Design review of the part built by this model. Coordinates are the model's own, in mm. Give positions to 0.01 mm unless a question says otherwise; leave off trailing zeros. Loops run counter-clockwise (first coordinate to the right, second up) from the corner with the lowest first, then second, coordinate; pieces in that order, holes last. Notation, with made-up numbers: M 17,36 L 57,36 A20 ccw 57,65 Z; hole C 28,-15 d9. An arc over 180 degrees is marked long. Use a Markdown table: item, result. Add a question column.
(1) Add section A-A, the plane x = -54.5. Give the boundary of the cut face in (y, z), then the cut area to 3 significant figures.
(2) Add section D-D, the plane x = -22. Give the boundary of the cut face in (y, z), then the cut area to 3 significant figures.
(3) Insertion check: pin 1 Ø0.9 at (y, z) = (-124.5, 2) entering from +X; pin 2 Ø0.9 at (x, z) = (-56, 2) entering from +Y; pin 3 Ø1.5 at (x, z) = (-42, 2) entering from -Y. Each pin has a flat end and moves straight along its axis. Give the tip position at first contact, or say it passes through.
(4) For probe 1 along Y at (x, z) = (16.5, 2.2); probe 2 along Y at (x, z) = (-44, 2.15); probe 3 along X at (y, z) = (53.5, 0.35), list the stretches that pass through material, from the lowest coordinate up.
(5) Add section B-B, the plane z = 2.2. State how many separate pieces and enclosed holes the cut face has, then the cut area to 3 significant figures.
(6) Add section C-C, the plane y = -28. Give the boundary of the cut face in (x, z).
Autodesk Fusion 360 part; units mm, degrees
sketch "Skizze1" plane through (0, 0, 0) normal (0, 0, 1) x (1, 0, 0)
  line L0 (-48.5045, 60.0252) -> (-48.5045, -50)
  line L1 (21.4307, 60.0126) -> (21.4307, -50)
  line L2 (-41.5077, 135.8568) -> (-13.5563, 144.0233)
  line L3 (-13.5563, 144.0233) -> (14.4793, 135.8568)
  line L4 (-41.4821, -125.8001) -> (-13.5254, -133.9377)
  line L5 (-13.5254, -133.9377) -> (14.4312, -125.8001)
  line L6 (14.4312, -125.8001) -> (14.4312, -57)
  line L7 (-41.4821, -125.8001) -> (-41.4821, -57)
  line L8 (-41.5077, 135.8568) -> (-41.5077, 66.6867)
  line L9 (14.4793, 135.8568) -> (14.4793, 66.6867)
  circle A0 centre (3.4202, 136.0177) radius 1.7651
  circle A1 centre (-30.4724, 136.0177) radius 1.7717
  circle A2 centre (-30.5621, -125.8912) radius 1.7405
  circle A3 centre (3.437, -125.8912) radius 1.7197
  circle A4 centre (-43.5796, -44.9629) radius 1.7343
  circle A5 centre (16.4191, -44.9629) radius 1.761
  circle A6 centre (-43.5796, 55.0289) radius 1.7075
  circle A7 centre (16.4191, 55.0289) radius 1.7507
  line L10 (21.4307, 60.0126) -> (21.4793, 60.0126)
  line L11 (14.4793, 67.0126) -> (14.4793, 66.6867)
  line L12 (-41.5077, 66.6867) -> (-41.5077, 67.0252)
  line L13 (-48.5077, 60.0252) -> (-48.5045, 60.0252)
  line L14 (-48.5045, -50) -> (-48.4821, -50)
  line L15 (21.4312, -50) -> (21.4307, -50)
  arc A8 (21.4312, -50) -> (14.4312, -57) centre (21.4312, -57) ccw
  arc A9 (-41.4821, -57) -> (-48.4821, -50) centre (-48.4821, -57) ccw
  arc A10 (-48.5077, 60.0252) -> (-41.5077, 67.0252) centre (-48.5077, 67.0252) ccw
  arc A11 (14.4793, 67.0126) -> (21.4793, 60.0126) centre (21.4793, 67.0126) ccw
  dimension "d1" = 7
  dimension "d2" = 7
  dimension "d3" = 7
  dimension "d4" = 7
extrude "Extrusion1" add sketch "Skizze1" along normal blind 3
sketch "Skizze2" plane through (0, 0, 3) normal (0, 0, 1) x (-1, 0, 0)
  circle A0 centre (43.5796, 44.9629) radius 1.7343
  circle A1 centre (30.5621, 125.8912) radius 1.7405
  circle A2 centre (-16.4191, -55.0289) radius 1.7507
  circle A3 centre (-16.4191, 44.9629) radius 1.761
  circle A4 centre (30.4724, -136.0177) radius 1.7717
  circle A5 centre (-3.437, 125.8912) radius 1.7197
  circle A6 centre (-3.4202, -136.0177) radius 1.7651
  circle A7 centre (43.5796, -55.0289) radius 1.7075
  line L0 (41.5077, -135.8568) -> (41.5077, -67.0252)
  arc A8 (48.5045, -60.0252) -> (41.5077, -67.0252) centre (48.5077, -67.0252) ccw
  line L1 (48.5045, -60.0252) -> (48.5045, 50)
  line L2 (48.5045, 50) -> (48.4821, 50)
  arc A9 (41.4821, 57) -> (48.4821, 50) centre (48.4821, 57) ccw
  line L3 (41.4821, 57) -> (41.4821, 125.8001)
  line L4 (41.4821, 125.8001) -> (13.5254, 133.9377)
  line L5 (13.5254, 133.9377) -> (-14.4312, 125.8001)
  line L6 (-14.4312, 125.8001) -> (-14.4312, 57)
  arc A10 (-21.4307, 50) -> (-14.4312, 57) centre (-21.4312, 57) ccw
  line L7 (-21.4307, 50) -> (-21.4307, -60.0126)
  line L8 (-21.4307, -60.0126) -> (-21.4793, -60.0126)
  arc A11 (-14.4793, -67.0126) -> (-21.4793, -60.0126) centre (-21.4793, -67.0126) ccw
  line L9 (-14.4793, -67.0126) -> (-14.4793, -135.8568)
  line L10 (-14.4793, -135.8568) -> (13.5563, -144.0233)
  line L11 (13.5563, -144.0233) -> (41.5077, -135.8568)
  line L12 (60.3895, -133.2143) -> (41.496, -133.2143)
  line L13 (41.496, -133.2143) -> (41.496, -60.1458)
  line L14 (60.3895, -60.1458) -> (60.3895, -133.2143)
  line L15 (-14.4793, -133.43) -> (-33.5, -133.43)
  line L16 (-33.5, -133.43) -> (-33.5, -60)
  line L17 (-33.5, -60) -> (-14.4793, -60)
  line L18 (-14.4793, -60) -> (-14.4793, -133.43)
  line L19 (60.4376, 49.7535) -> (40.5505, 49.7535)
  line L20 (40.5505, 49.7535) -> (40.5505, 122.7237)
  line L21 (40.5505, 122.7237) -> (60.4376, 122.7237)
  line L22 (60.4376, 122.7237) -> (60.4376, 49.7535)
  line L23 (-12.9102, 49.7535) -> (-33.4913, 49.7535)
  line L24 (-33.4913, 49.7535) -> (-33.4913, 122.7237)
  line L25 (-33.4913, 122.7237) -> (-12.9102, 122.7237)
  line L26 (-12.9102, 122.7237) -> (-12.9102, 49.7535)
sketch "Skizze3" plane through (0, 0, 3) normal (0, 0, 1) x (-1, 0, 0)
  line L0 (60.4211, -59.9543) -> (41.4063, -59.9543)
  line L1 (41.4063, -59.9543) -> (41.4063, -133.2514)
  line L2 (41.4063, -133.2514) -> (60.4211, -133.2514)
  line L3 (60.4211, -133.2514) -> (60.4211, -59.9543)
extrude "Extrusion2" add sketch "Skizze3" sketch "Skizze2" against normal blind 3 of sketch 2 contours L7 A11 L9 L15 L16 L17 L18 | L1 L2 A9 L3 L19 L21 L22 | L6 A10 L7 L23 L24 L25
Established:
| question | item | result |
|---|---|---|
| 1 | outline | M -122.72,0 L -49.75,0 L -49.75,3 L -122.72,3 Z; M 59.95,0 L 133.25,0 L 133.25,3 L 59.95,3 Z |
| 1 | area | 439 mm^2 |
| 2 | outline | M -131.47,0 L 141.56,0 L 141.56,3 L -131.47,3 Z |
| 2 | area | 819 mm^2 |
| 3 | pin 1 | x = 14.43 |
| 3 | pin 2 | y = 133.25 |
| 3 | pin 3 | y = -125.87 |
| 4 | probe 1 | -122.72 to -46.72, -43.2 to 53.28, 56.78 to 133.43 |
| 4 | probe 2 | -122.72 to -46.65, -43.28 to 53.37, 56.68 to 133.25 |
| 4 | probe 3 | -48.5 to -44.34, -42.82 to 15.57, 17.27 to 21.43 |
| 5 | separate pieces | 1 |
| 5 | enclosed holes | 8 |
| 5 | area | 22,100 mm^2 |
| 6 | outline | M -48.5,0 L 21.43,0 L 21.43,3 L -48.5,3 Z |
